Here's how the part is built. I have some questions about the finished solid (model axes, mm). A direction names the side the tool comes from. Round coordinates to 2 decimals unless told otherwise and drop trailing zeros. Write each loop counter-clockwise with the first axis right and the second up, starting at its lowest first coordinate (ties: lowest second). Pieces come first, ordered by that corner, then holes. Notation, with made-up numbers: (-32.75, 71.25) -> (-18.75, 71.25) arc R18 ccw to (-18.75, 96.25) -> close; hole circle Ø9 at (-28, -29). An arc over 180 degrees is marked (long way). Answer in a Markdown table with one row per item.
from build123d import *
from build123d import SkipClean  # not in build123d's __all__

# Parameters (mm, degrees)
F1_DEPTH = 19.05
F2_DEPTH = 0.635
F4_DEPTH = 0.635


with BuildPart() as f1:
    # F0 (on Front) → F1 (new body)
    with BuildSketch(Plane.XZ):
        with BuildLine():
            Line((7.6934193521, 67.6337401125), (-10.4047286745, 67.6337401125))
            Line((-10.4047286745, 67.6337401125), (-10.4047286745, 16.8337401125))
            Line((-10.4047286745, 16.8337401125), (7.6934193521, 16.8337401125))
            ThreePointArc((7.6934193521, 16.8337401125), (10.8042713255, 17.4687401125), (13.9151232988, 16.8337401125))
            Line((13.9151232988, 16.8337401125), (32.0132713255, 16.8337401125))
            Line((32.0132713255, 16.8337401125), (32.0132713255, 67.6337401125))
            Line((32.0132713255, 67.6337401125), (13.9151232988, 67.6337401125))
            ThreePointArc((13.9151232988, 67.6337401125), (10.8042713255, 66.9987401125), (7.6934193521, 67.6337401125))
        make_face()
    extrude(amount=F1_DEPTH)

    # F0 (on Front) → F2 (join)
    with BuildSketch(Plane.XZ):
        with BuildLine():
            ThreePointArc((32.0132713255, 67.6337401125), (10.8042713255, 88.8427401125), (-10.4047286745, 67.6337401125))
            Line((-10.4047286745, 67.6337401125), (7.6934193521, 67.6337401125))
            ThreePointArc((7.6934193521, 67.6337401125), (6.4275420266, 81.5580334417), (18.7417713255, 74.9362401125))
            ThreePointArc((18.7417713255, 74.9362401125), (17.4260646546, 70.5595108136), (13.9151232988, 67.6337401125))
            Line((13.9151232988, 67.6337401125), (32.0132713255, 67.6337401125))
        make_face()
        with BuildLine():
            Line((7.6934193521, 67.6337401125), (-10.4047286745, 67.6337401125))
            Line((-10.4047286745, 67.6337401125), (-10.4047286745, 16.8337401125))
            Line((-10.4047286745, 16.8337401125), (7.6934193521, 16.8337401125))
            ThreePointArc((7.6934193521, 16.8337401125), (10.8042713255, 17.4687401125), (13.9151232988, 16.8337401125))
            Line((13.9151232988, 16.8337401125), (32.0132713255, 16.8337401125))
            Line((32.0132713255, 16.8337401125), (32.0132713255, 67.6337401125))
            Line((32.0132713255, 67.6337401125), (13.9151232988, 67.6337401125))
            ThreePointArc((13.9151232988, 67.6337401125), (10.8042713255, 66.9987401125), (7.6934193521, 67.6337401125))
        make_face()
        with BuildLine():
            Line((7.6934193521, 16.8337401125), (-10.4047286745, 16.8337401125))
            ThreePointArc((-10.4047286745, 16.8337401125), (10.8042713255, -4.3752598875), (32.0132713255, 16.8337401125))
            Line((32.0132713255, 16.8337401125), (13.9151232988, 16.8337401125))
            ThreePointArc((13.9151232988, 16.8337401125), (17.4260646546, 13.9079694114), (18.7417713255, 9.5312401125))
            ThreePointArc((18.7417713255, 9.5312401125), (6.4275420266, 2.9094467834), (7.6934193521, 16.8337401125))
        make_face()
    extrude(amount=F2_DEPTH)

    # F3 (on face) → F4 (join)
    with BuildSketch(Plane.XZ.offset(19.05)):
        with BuildLine():
            ThreePointArc((-10.4047286745, 16.8337401125), (10.8042713255, -4.3752598875), (32.0132713255, 16.8337401125))
            Line((32.0132713255, 16.8337401125), (13.9151232988, 16.8337401125))
            ThreePointArc((13.9151232988, 16.8337401125), (17.4260646546, 13.9079694114), (18.7417713255, 9.5312401125))
            ThreePointArc((18.7417713255, 9.5312401125), (6.4275420266, 2.9094467834), (7.6934193521, 16.8337401125))
            Line((7.6934193521, 16.8337401125), (-10.4047286745, 16.8337401125))
        make_face()
        with BuildLine():
            Line((13.9151232988, 67.6337401125), (32.0132713255, 67.6337401125))
            ThreePointArc((32.0132713255, 67.6337401125), (10.8042713255, 88.8427401125), (-10.4047286745, 67.6337401125))
            Line((-10.4047286745, 67.6337401125), (7.6934193521, 67.6337401125))
            ThreePointArc((7.6934193521, 67.6337401125), (6.4275420266, 81.5580334417), (18.7417713255, 74.9362401125))
            ThreePointArc((18.7417713255, 74.9362401125), (17.4260646546, 70.5595108136), (13.9151232988, 67.6337401125))
        make_face()
    with SkipClean():  # cleaning this boolean's faces spoils the solid; the shape is the same uncleaned
        extrude(amount=-F4_DEPTH)


solid = f1.part
1) I want a section at B-B, the plane z = 71.5. List the corners of the cut face in (x, y) for me (3 decimals), and give its area (3 significant figures).
Response:
| item | result |
|---|---|
| outline | (-10.049, -19.05) -> (3.649, -19.05) -> (3.649, -18.415) -> (-10.049, -18.415) -> close; (-10.049, -0.635) -> (3.649, -0.635) -> (3.649, 0) -> (-10.049, 0) -> close; (17.959, -19.05) -> (31.658, -19.05) -> (31.658, -18.415) -> (17.959, -18.415) -> close; (17.959, -0.635) -> (31.658, -0.635) -> (31.658, 0) -> (17.959, 0) -> close |
| area | 34.8 mm^2 |
2) I need wall thicknesses on line 1 (Y direction, x = -4, z = 76.5) (3 decimals); line 2 (Z direction, x = 26, y = -13.25); line 3 (Z direction, x = 13, y = -16.75). Which ranges of each line are inside material? Lowest first, please. Write a range as [from, to].
Response:
| item | result |
|---|---|
| line 1 | y = [-19.05, -18.415], [-0.635, 0] |
| line 2 | z = [16.83, 67.63] |
| line 3 | z = [17.16, 67.31] |
3) I want a section at D-D, the plane x = 5.5. List the corners of the cut face in (y, z) for me (3 decimals).
Response:
| item | result |
|---|---|
| outline | (-19.05, -3.701) -> (-18.415, -3.701) -> (-18.415, 3.626) -> (-19.05, 3.626) -> close; (-19.05, 15.436) -> (-18.415, 15.436) -> (-18.415, 16.834) -> (-0.635, 16.834) -> (-0.635, 15.436) -> (0, 15.436) -> (0, 69.031) -> (-0.635, 69.031) -> (-0.635, 67.634) -> (-18.415, 67.634) -> (-18.415, 69.031) -> (-19.05, 69.031) -> close; (-19.05, 80.841) -> (-18.415, 80.841) -> (-18.415, 88.169) -> (-19.05, 88.169) -> close; (-0.635, -3.701) -> (0, -3.701) -> (0, 3.626) -> (-0.635, 3.626) -> close; (-0.635, 80.841) -> (0, 80.841) -> (0, 88.169) -> (-0.635, 88.169) -> close |
4) We'd pull the mould along Y, two halves only. Please class faces 1 (the face through (-10.405, -9, 43)), 2 (the face through (11, -19.05, 43)), 3 (the face through (23, -9, 16.834)): +Y half, -Y half, draft (parallel to the pull), parting line (faces both ways), or undercut.
Response:
| item | result |
|---|---|
| face 1 | draft |
| face 2 | -Y half |
| face 3 | undercut |
5) I want a section at C-C, the plane y = -8.5. List the corners of the cut face in (x, z) for me (1 decimal), and give its area (3 significant figures).
Response:
| item | result |
|---|---|
| outline | (-10.4, 16.8) -> (7.7, 16.8) arc R7.9 cw to (13.9, 16.8) -> (32, 16.8) -> (32, 67.6) -> (13.9, 67.6) arc R7.9 cw to (7.7, 67.6) -> (-10.4, 67.6) -> close |
| area | 2,150 mm^2 |
6) Which directions (+Z, -Z, +X, -X, +Y, -Y) give clear straight access to the entire face, cutting with the end or side of a thin tool? Please do faces 4 (the face through (23, -9, 67.634)), 5 (the face through (10.34, -0.31, -4.37)), 6 (the face through (6, -0.635, 2)).
Response:
| item | result |
|---|---|
| face 4 | +Z, +X, -X |
| face 5 | -Z, +Y, -Y |
| face 6 | -Z, +X, -X |
7) For pin 1 (14.5 mm diameter, centred on x = 10.8, z = 74.94, fed in from +Y); pin 2 (5.5 mm diameter, centred on x = 24.5, y = -12.5, fed in from +Z), each with a flat end and sliding along its axis, tell me the tip position at first contact or that it passes through.
Response:
| item | result |
|---|---|
| pin 1 | passes through |
| pin 2 | stops at z = 67.63 |
8) I want a section at A-A, the plane x = 16.5. List the corners of the cut face in (y, z) for me (3 decimals), and give its area (3 significant figures).
Response:
| item | result |
|---|---|
| outline | (-19.05, -3.596) -> (-18.415, -3.596) -> (-18.415, 4.003) -> (-19.05, 4.003) -> close; (-19.05, 15.06) -> (-18.415, 15.06) -> (-18.415, 16.834) -> (-0.635, 16.834) -> (-0.635, 15.06) -> (0, 15.06) -> (0, 69.408) -> (-0.635, 69.408) -> (-0.635, 67.634) -> (-18.415, 67.634) -> (-18.415, 69.408) -> (-19.05, 69.408) -> close; (-19.05, 80.465) -> (-18.415, 80.465) -> (-18.415, 88.064) -> (-19.05, 88.064) -> close; (-0.635, -3.596) -> (0, -3.596) -> (0, 4.003) -> (-0.635, 4.003) -> close; (-0.635, 80.465) -> (0, 80.465) -> (0, 88.064) -> (-0.635, 88.064) -> close |
| area | 992 mm^2 |
